```python
from build123d import *

# Parameters (mm, degrees)
SKETCH_1_W      = 82
SKETCH_1_H      = 101
SKETCH_1_R      = 1.55
EXTRUDE_1_DEPTH = 3
FILLET_1_R      = 5


with BuildPart() as part:
    # 草图1 → 凸台-拉伸1 (new body)
    with BuildSketch(Plane.XY):
        with Locations((41, 50.5)):
            Rectangle(SKETCH_1_W, SKETCH_1_H)
        with Locations((41, 6)):
            Circle(SKETCH_1_R, mode=Mode.SUBTRACT)
        with Locations((66, 6)):
            Circle(SKETCH_1_R, mode=Mode.SUBTRACT)
        with Locations((16, 6)):
            Circle(SKETCH_1_R, mode=Mode.SUBTRACT)
        with Locations((41, 95)):
            Circle(SKETCH_1_R, mode=Mode.SUBTRACT)
        with Locations((66, 95)):
            Circle(SKETCH_1_R, mode=Mode.SUBTRACT)
        with Locations((16, 95)):
            Circle(SKETCH_1_R, mode=Mode.SUBTRACT)
    extrude(amount=EXTRUDE_1_DEPTH)

    # 圆角1
    fillet_1_edges = [part.edges().sort_by_distance(p)[0] for p in [
        (0, 101, 1.5),
        (82, 101, 1.5),
        (82, 0, 1.5),
        (0, 0, 1.5),
    ]]
    fillet(fillet_1_edges, radius=FILLET_1_R)


solid = part.part
```
Can you work these out from the model? Positions are in its coordinate system, mm. Coordinates: 2 decimals unless noted, no trailing zeros. Loops run counter-clockwise (first coordinate to the right, second up) from the corner with the lowest first, then second, coordinate; pieces in that order, holes last. Notation, with made-up numbers: (32, 26) -> (61, 26) arc R28 ccw to (61, 55) -> close; hole circle Ø9 at (23, 72.5). An arc over 180 degrees is marked (long way). Put each result on its own line as item: value. Start each with the question number.
Q1. I want a section at A-A (x = 41). Write out the boundary of the cut face in (y, z), plus the area to 3 significant figures.
Q2. Thinking about a two-plate mould opening in X: for faces 1 (the face through (42.478, 6.466, 1.479)), 2 (the face through (82, 50, 1)), 3 (the face through (1, 99, 2)), which applies, pulls with the +X half, pulls with the -X half, needs draft (parallel to the pull), parting line crosses it, or undercut?
Q3. If I drill on line 1 (Y direction, x = 66, z = 1.5); line 2 (X direction, y = 95, z = 1.6); line 3 (X direction, y = 7, z = 1.7), over which ranges is the centre line in solid material (lowest first)? Write a range as [from, to].
Taken from the geometry:
1. outline: (0, 0) -> (4.45, 0) -> (4.45, 3) -> (0, 3) -> close; (7.55, 0) -> (93.45, 0) -> (93.45, 3) -> (7.55, 3) -> close; (96.55, 0) -> (101, 0) -> (101, 3) -> (96.55, 3) -> close
1. area: 284 mm2
2. face 1: undercut
2. face 2: pulls with the +X half
2. face 3: pulls with the -X half
3. line 1: y = [0, 4.45], [7.55, 93.45], [96.55, 101]
3. line 2: x = [0, 14.45], [17.55, 39.45], [42.55, 64.45], [67.55, 82]
3. line 3: x = [0, 14.82], [17.18, 39.82], [42.18, 64.82], [67.18, 82]
